Geometry check sheet. Reference: the model listing, model coordinates, mm. Round coordinates to 2 decimals unless told otherwise and drop trailing zeros. Write each loop counter-clockwise with the first axis right and the second up, starting at its lowest first coordinate (ties: lowest second). Pieces come first, ordered by that corner, then holes. Notation, with made-up numbers: M -27.5,72.25 L 21.5,72.25 A9 ccw 21.5,86.25 Z; hole C -27,27 d11. An arc over 180 degrees is marked long. Use a Markdown table: item, result.
```python
from build123d import *

# Parameters (mm, degrees)
BOSS_EXTRUDE1_DEPTH         = 355.6
F_27_0_144_DIAMETER_HOLE1_D = 2.100000118


with BuildPart() as part:
    # Sketch1 → Boss-Extrude1 (new body)
    with BuildSketch(Plane(origin=(0, 0, 0), x_dir=(1, 0, 0), z_dir=(0, 1, 0))):
        Polygon((-24.676553482, 0), (-24.676553482, -25.4), (-11.976553482, -25.4), (-11.976553482, -16.933333333), (-4.644205064, -21.166666667), (-4.644205064, -4.233333333), (-11.976553482, -8.466666667), (-11.976553482, 0), align=None)
    extrude(amount=BOSS_EXTRUDE1_DEPTH)

    # #27 (0.144) Diameter Hole1 (through all)
    with Locations(Plane(origin=(0, 0, 0), x_dir=(-1, 0, 0), z_dir=(0, 0, -1))):
        with Locations((18.879197864, 341.956469662), (18.879197864, 329.626469662), (18.879197864, 317.180469662), (18.879197864, 304.734469662), (18.879197864, 292.288469662), (18.879197864, 279.842469662), (18.879197864, 267.396469662), (18.879197864, 254.950469662), (18.879197864, 242.504469662), (18.879197864, 230.058469662), (18.879197864, 217.612469662), (18.879197864, 205.166469662), (18.879197864, 192.720469662), (18.879197864, 179.588809686), (18.879197864, 167.828469662), (18.879197864, 155.382469662), (18.879197864, 142.936469662), (18.879197864, 130.490469662), (18.879197864, 118.044469662), (18.879197864, 105.598469662), (18.879197864, 93.152469662), (18.879197864, 80.706469662), (18.879197864, 68.260469662), (18.879197864, 55.814469662), (18.879197864, 43.368469662), (18.879197864, 30.922469662), (18.879197864, 18.476469662), (18.879197864, 6.030469662)):
            Hole(F_27_0_144_DIAMETER_HOLE1_D / 2)


solid = part.part
```
Item 1: Material ranges on line 1 along X through (y, z) = (143.5, 8.75); line 2 along X through (y, z) = (43, 11.25); line 3 along X through (y, z) = (43, 4.75), recorded low to high. Write a range as from..to.
Outcome:
| item | result |
|---|---|
| line 1 | x = -24.68..-19.77, -17.99..-4.64 |
| line 2 | x = -24.68..-19.86, -17.9..-4.64 |
| line 3 | x = -24.68..-19.86, -17.9..-11.98, -5.54..-4.64 |
Item 2: Mould release check, pull along X, two halves, no side actions. Record for faces 1 (the face through (-11.977, 175, 21)), 2 (the face through (-4.644, 175, 13)), 3 (the face through (-18, 175, 0)), 4 (the face through (-24.677, 175, 13)): +X half, -X half, draft (parallel to the pull), parting line (faces both ways), or undercut.
Outcome:
| item | result |
|---|---|
| face 1 | undercut |
| face 2 | +X half |
| face 3 | draft |
| face 4 | -X half |
Item 3: Go/stop test with a flat-tipped pin: pin 1 (3.5 mm diameter, centred on x = -18.88, y = 254.95, fed in from +Z). Record where the tip stops, or that it passes through.
Outcome:
| item | result |
|---|---|
| pin 1 | stops at z = 25.4 |
Item 4: Cross-section at A-A, the plane y = 149.5. Record the cut outline in (x, z), and give its area (3 significant figures).
Outcome:
| item | result |
|---|---|
| outline | M -24.68,0 L -11.98,0 L -11.98,8.47 L -4.64,4.23 L -4.64,21.17 L -11.98,16.93 L -11.98,25.4 L -24.68,25.4 Z |
| area | 416 mm2 |
